Study the drawing (mm; zero at the part's minimum x, y, z) and answer. Coordinates: 2 decimals unless noted, no trailing zeros. Order: outer loops, then holes, each group sorted by start corner. A loop starts at its lowest first (then second) coordinate and runs counter-clockwise, first axis right, second up. Notation, with made-up numbers: M -33,-15 L -3,-15 A16 cw -3,4 Z; hole C -34.75,18 d3. An arc over 180 degrees is marked long. One line per item, written item: value. Start each with the question number.
Q1. This flat-tipped pin is pushed along its axis until it touches: pin 1 Ø6 at (x, y) = (13, 30.5) entering from -Z. Where does it stop, or does it pass through?
Q2. Straight lines are drawn through the part: line 1 along X through (y, z) = (25, 0.3); line 2 along Y through (x, z) = (13, 0.1); line 3 along Y through (x, z) = (8.5, 0.3). For each, find the intervals that lie inside material, in ascending order. Write a range as [from, to].
Q3. The part is cut by section D-D on y = 5. Give the vertices of the cut face in (x, z).
Q4. The part is cut by section C-C on z = 0.25. Give the vertices of the cut face in (x, y).
Q5. The part is cut by section A-A on y = 23. Give the vertices of the cut face in (x, z), then the cut area to 3 significant figures.
Q6. The part is cut by section B-B on x = 12.5. Give the vertices of the cut face in (y, z).
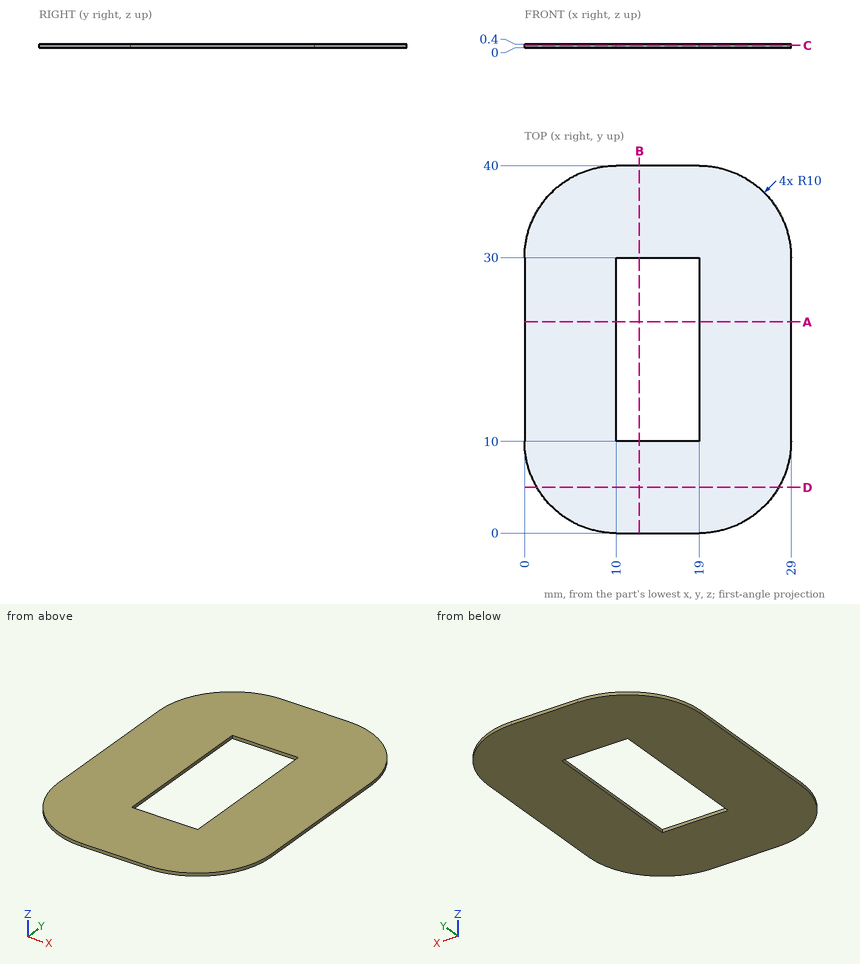
Output:
1. pin 1: stops at z = 0
2. line 1: x = [0, 10], [19, 29]
2. line 2: y = [0, 10], [30, 40]
2. line 3: y = [0.11, 39.89]
3. outline: M 1.34,0 L 27.66,0 L 27.66,0.4 L 1.34,0.4 Z
4. outline: M 0,10 A10 ccw 10,0 L 19,0 A10 ccw 29,10 L 29,30 A10 ccw 19,40 L 10,40 A10 ccw 0,30 Z; hole M 10,10 L 19,10 L 19,30 L 10,30 Z
5. outline: M 0,0 L 10,0 L 10,0.4 L 0,0.4 Z; M 19,0 L 29,0 L 29,0.4 L 19,0.4 Z
5. area: 8.00 mm^2
6. outline: M 0,0 L 10,0 L 10,0.4 L 0,0.4 Z; M 30,0 L 40,0 L 40,0.4 L 30,0.4 Z
